Read the model definition and answer for the solid it produces. Units are mm, in the model's axes. A direction names the side the tool comes from. Coordinates: 2 decimals unless noted, no trailing zeros. Loops run counter-clockwise (first coordinate to the right, second up) from the corner with the lowest first, then second, coordinate; pieces in that order, holes last. Notation, with made-up numbers: (76.25, 21) -> (113.25, 21) arc R8 cw to (113.25, 25) -> close; hole circle Ø5 at (33.25, 7.25). An arc over 180 degrees is marked (long way). Answer as a JSON object with one key per item and string values. Group by question number.
1) Flat-ended cylindrical pins translate along their axes: P1, Ø1, axis at x = 28.5, z = 740, coming from the -Y side; P2, Ø5, axis at x = 11, z = 705.5, coming from the +Y side; P3, Ø24, axis at y = 45, z = 708, coming from the +X side; P4, Ø10, axis at x = 35.5, z = 658, coming from the +Y side. Find the tip coordinate at first contact, or state that the pin passes through.
2) Which of the six approach directions +Z, -Z, +X, -X, +Y, -Y give full straight-line access (tool end or side, diameter ignored) to faces 1 (the face through (6, 20, 0)), 2 (the face through (36, 6.35, 582))?
3) Section A-A, the plane z = 336.5 is taken. Give the vertices of the cut face in (x, y) (3 decimals), plus the area to 3 significant figures.
4) Consider probe 1 along X at (y, z) = (40, 817); probe 2 along X at (y, z) = (11.5, 819). Determine where each line is inside the solid, lowest interval first. Write a range as [from, to].
5) Section B-B, the plane x = 39 is taken. Give the vertices of the cut face in (y, z).
Autodesk Inventor part; units mm, degrees
ref_plane "YZ Plane" through (0, 0, 0) normal (1, 0, 0) x (0, 1, 0)
ref_plane "XZ Plane" through (0, 0, 0) normal (0, 1, 0) x (-1, 0, 0)
ref_plane "XY Plane" through (0, 0, 0) normal (0, 0, 1) x (1, 0, 0)
sketch "Sketch1" plane through (0, 0, 0) normal (0, 0, 1) x (1, 0, 0)
  line L0 (0, 0) -> (0, 63.5)
  line L1 (0, 63.5) -> (3.175, 63.5)
  line L2 (6.35, 60.325) -> (6.35, 12.7)
  line L3 (12.7, 6.35) -> (60.325, 6.35)
  line L4 (63.5, 3.175) -> (63.5, 0)
  line L5 (63.5, 0) -> (0, 0)
  arc A0 (6.35, 12.7) -> (12.7, 6.35) centre (12.7, 12.7) ccw
  arc A1 (63.5, 3.175) -> (60.325, 6.35) centre (60.325, 3.175) ccw
  arc A2 (6.35, 60.325) -> (3.175, 63.5) centre (3.175, 60.325) ccw
  dimension "d0" = 63.5
  dimension "d1" = 6.35
  dimension "d2" = 6.35
  dimension "d3" = 3.175
extrude "Extrusion1" add sketch "Sketch1" along normal blind 1181.1
properties part number "GE-12019-06" material "Aluminum-6061"
Determined:
{
 "1": {"P1": "y = 0", "P2": "y = 7.94", "P3": "x = 6.35", "P4": "y = 6.35"},
 "2": {"face 1": "-Z, +X, -X, +Y, -Y", "face 2": "+Z, -Z, +X, +Y"},
 "3": {"outline": "(0, 0) -> (63.5, 0) -> (63.5, 3.175) arc R3.175 ccw to (60.325, 6.35) -> (12.7, 6.35) arc R6.35 cw to (6.35, 12.7) -> (6.35, 60.325) arc R3.175 ccw to (3.175, 63.5) -> (0, 63.5) -> close", "area": "770 mm²"},
 "4": {"probe 1": "[0, 6.35]", "probe 2": "[0, 6.46]"},
 "5": {"outline": "(0, 0) -> (6.35, 0) -> (6.35, 1181.1) -> (0, 1181.1) -> close"}
}
